Model file for the job. Use its own axes, mm. Coordinates: 2 decimals unless noted, no trailing zeros. Loops run counter-clockwise (first coordinate to the right, second up) from the corner with the lowest first, then second, coordinate; pieces in that order, holes last.
from build123d import *

# Parameters (mm, degrees)
F0_R     = 76.2
F0_R_2   = 4.7625
F1_DEPTH = 25.4
F2_R     = 6.35


with BuildPart() as f1:
    # F0 (on Front) → F1 (new body)
    with BuildSketch(Plane.XZ):
        Circle(F0_R)
        with BuildLine():
            ThreePointArc((66.504693, 4.7625), (66.63241, 2.382772), (66.675, 0))
            ThreePointArc((66.675, 0), (66.63241, -2.382772), (66.504693, -4.7625))
            ThreePointArc((66.504693, -4.7625), (47.146345, -47.146345), (4.7625, -66.504693))
            ThreePointArc((4.7625, -66.504693), (0, -66.675), (-4.7625, -66.504693))
            ThreePointArc((-4.7625, -66.504693), (-47.146345, -47.146345), (-66.504693, -4.7625))
            ThreePointArc((-66.504693, -4.7625), (-66.675, 0), (-66.504693, 4.7625))
            ThreePointArc((-66.504693, 4.7625), (-47.146345, 47.146345), (-4.7625, 66.504693))
            ThreePointArc((-4.7625, 66.504693), (0, 66.675), (4.7625, 66.504693))
            ThreePointArc((4.7625, 66.504693), (47.146345, 47.146345), (66.504693, 4.7625))
        make_face(mode=Mode.SUBTRACT)
        with BuildLine():
            Line((4.7625, 18.445083), (4.7625, 66.504693))
            ThreePointArc((4.7625, 66.504693), (0, 66.675), (-4.7625, 66.504693))
            Line((-4.7625, 66.504693), (-4.7625, 18.445083))
            ThreePointArc((-4.7625, 18.445083), (0, 19.05), (4.7625, 18.445083))
        make_face()
        with BuildLine():
            ThreePointArc((66.504693, -4.7625), (66.63241, -2.382772), (66.675, 0))
            ThreePointArc((66.675, 0), (66.63241, 2.382772), (66.504693, 4.7625))
            Line((66.504693, 4.7625), (18.445083, 4.7625))
            ThreePointArc((18.445083, 4.7625), (18.898166, 2.400382), (19.05, 0))
            ThreePointArc((19.05, 0), (18.898166, -2.400382), (18.445083, -4.7625))
            Line((18.445083, -4.7625), (66.504693, -4.7625))
        make_face()
        with BuildLine():
            ThreePointArc((19.05, 0), (18.898166, 2.400382), (18.445083, 4.7625))
            ThreePointArc((18.445083, 4.7625), (13.470384, 13.470384), (4.7625, 18.445083))
            ThreePointArc((4.7625, 18.445083), (0, 19.05), (-4.7625, 18.445083))
            ThreePointArc((-4.7625, 18.445083), (-13.470384, 13.470384), (-18.445083, 4.7625))
            ThreePointArc((-18.445083, 4.7625), (-19.05, 0), (-18.445083, -4.7625))
            ThreePointArc((-18.445083, -4.7625), (-13.470384, -13.470384), (-4.7625, -18.445083))
            ThreePointArc((-4.7625, -18.445083), (0, -19.05), (4.7625, -18.445083))
            ThreePointArc((4.7625, -18.445083), (13.470384, -13.470384), (18.445083, -4.7625))
            ThreePointArc((18.445083, -4.7625), (18.898166, -2.400382), (19.05, 0))
        make_face()
        Circle(F0_R_2, mode=Mode.SUBTRACT)
        with BuildLine():
            ThreePointArc((-4.7625, -66.504693), (0, -66.675), (4.7625, -66.504693))
            Line((4.7625, -66.504693), (4.7625, -18.445083))
            ThreePointArc((4.7625, -18.445083), (0, -19.05), (-4.7625, -18.445083))
            Line((-4.7625, -18.445083), (-4.7625, -66.504693))
        make_face()
        with BuildLine():
            Line((-18.445083, 4.7625), (-66.504693, 4.7625))
            ThreePointArc((-66.504693, 4.7625), (-66.675, 0), (-66.504693, -4.7625))
            Line((-66.504693, -4.7625), (-18.445083, -4.7625))
            ThreePointArc((-18.445083, -4.7625), (-19.05, 0), (-18.445083, 4.7625))
        make_face()
    extrude(amount=F1_DEPTH)

    # F2
    f2_edges = [f1.edges().sort_by_distance(p)[0] for p in [
        (4.7625, -12.7, 18.445083),
        (18.445083, -12.7, 4.7625),
        (-66.504693, -12.7, 4.7625),
        (4.7625, -12.7, -66.504693),
        (-18.445083, -12.7, 4.7625),
        (-4.7625, -12.7, 18.445083),
        (-4.7625, -12.7, -66.504693),
        (66.504693, -12.7, 4.7625),
        (18.445083, -12.7, -4.7625),
        (4.7625, -12.7, -18.445083),
        (4.7625, -12.7, 66.504693),
        (-66.504693, -12.7, -4.7625),
        (-4.7625, -12.7, -18.445083),
        (-18.445083, -12.7, -4.7625),
        (-4.7625, -12.7, 66.504693),
        (66.504693, -12.7, -4.7625),
    ]]
    fillet(f2_edges, radius=F2_R)


solid = f1.part
Q1. Slice it at D-D (z = 30.5). List the corners of the cut face in (x, y).
Answers:
outline: (-69.83, -25.4) - (-59.29, -25.4) - (-59.29, 0) - (-69.83, 0) - close; (-4.76, -25.4) - (4.76, -25.4) - (4.76, 0) - (-4.76, 0) - close; (59.29, -25.4) - (69.83, -25.4) - (69.83, 0) - (59.29, 0) - close
Q2. Slice it at C-C (y = -15.5). Count the separate pieces of the cut face and the enclosed holes in it, and give its area (3 significant figures).
Answers:
separate pieces: 1
enclosed holes: 5
area: 7,290 mm2
Q3. Mould opens along Z. For faces 1 (the flat face through (16, 0, 1)), 2 (the cylindrical face through (7.12, -12.88, -64.23)), 3 (the cylindrical face through (-60.47, -12.522, -46.367)) say: +Z half, -Z half, draft (parallel to the pull), parting line (faces both ways), or undercut.
Answers:
face 1: draft
face 2: undercut
face 3: parting line
Q4. Slice it at A-A (z = 0). List the corners of the cut face in (x, y), and give its area (3 significant figures).
Answers:
outline: (-76.2, -25.4) - (-4.76, -25.4) - (-4.76, 0) - (-76.2, 0) - close; (4.76, -25.4) - (76.2, -25.4) - (76.2, 0) - (4.76, 0) - close
area: 3,630 mm2
Q5. Slice it at B-B (x = 0). List the corners of the cut face in (y, z).
Answers:
outline: (-25.4, -76.2) - (0, -76.2) - (0, -4.76) - (-25.4, -4.76) - close; (-25.4, 4.76) - (0, 4.76) - (0, 76.2) - (-25.4, 76.2) - close
Q6. Flat gauge pins, fed straight in: P1, Ø3, axis at y = -4, z = -9, coming from the -X side; P2, Ø5, axis at x = -27, y = -4, coming from the -Z side; P3, Ø6, axis at y = -7, z = 29.5, coming from the -X side. Where does each tip first touch, or does it go through?
Answers:
P1: stops at x = -75.83
P2: stops at z = -72.15
P3: stops at x = -71.44
Q7. Drill centre lines: line 1 (X direction, y = -23.25, z = -13.5); line 2 (X direction, y = -22.25, z = 51.5); line 3 (Z direction, x = 17.5, y = -7.5). Where is each one in solid material? Low to high.
Answers:
line 1: x = -74.99 to -65.29, -13.44 to 13.44, 65.29 to 74.99
line 2: x = -56.16 to -42.35, -4.76 to 4.76, 42.35 to 56.16
line 3: z = -74.16 to -64.34, -7.68 to 7.68, 64.34 to 74.16
